Design review of the part built by this model. Coordinates are the model's own, in mm. A direction names the side the tool comes from. Give positions to 0.01 mm unless a question says otherwise; leave off trailing zeros. Write each loop counter-clockwise with the first axis right and the second up, starting at its lowest first coordinate (ties: lowest second). Pieces come first, ordered by that corner, then holes. Notation, with made-up numbers: (36, -38) - (90, -38) arc R11 cw to (90, -28) - close; hole circle Ø6 at (-37.75, 57). An arc over 180 degrees is marked (long way). Use a Markdown table: item, result. Add a question column.
```python
from build123d import *

# Parameters (mm, degrees)
SKETCH1_W           = 61
SKETCH1_H           = 61
SKETCH1_W_2         = 57
SKETCH1_H_2         = 57
BOSS_EXTRUDE2_DEPTH = 30
SKETCH2_W           = 58.6
SKETCH2_H           = 58.6
CUT_EXTRUDE1_DEPTH  = 3.2
SKETCH4_RX          = 3
SKETCH4_RY          = 2.5
CUT_EXTRUDE2_DEPTH  = 73.878323252
SKETCH5_W           = 57
SKETCH5_H           = 57
BOSS_EXTRUDE3_DEPTH = 2


with BuildPart() as part:
    # Sketch1 → Boss-Extrude2 (new body)
    with BuildSketch(Plane(origin=(0, 0, 0), x_dir=(1, 0, 0), z_dir=(0, 1, 0))):
        with Locations((0, 28.5)):
            Rectangle(SKETCH1_W, SKETCH1_H)
        with Locations((0, 28.5)):
            Rectangle(SKETCH1_W_2, SKETCH1_H_2, mode=Mode.SUBTRACT)
    extrude(amount=BOSS_EXTRUDE2_DEPTH)

    # Sketch2 → Cut-Extrude1 (cut)
    with BuildSketch(Plane(origin=(0, 30, 0), x_dir=(1, 0, 0), z_dir=(0, 1, 0))):
        with Locations((0, 28.5)):
            Rectangle(SKETCH2_W, SKETCH2_H)
    extrude(amount=-CUT_EXTRUDE1_DEPTH, mode=Mode.SUBTRACT)

    # Sketch4 → Cut-Extrude2 (cut, through all)
    with BuildSketch(Plane(origin=(0, 0, 0), x_dir=(-1, 0, 0), z_dir=(0, 0, -1))):
        with BuildLine():
            Line((-5.98277454, 23.2), (-5.98277454, 25.8))
            Line((-5.98277454, 25.8), (-8.131556664, 25.8))
            ThreePointArc((-8.131556664, 25.8), (-8.523646049, 25.719927124), (-8.852943985, 25.492531828))
            Line((-8.852943985, 25.492531828), (-9.479161861, 24.840221541))
            ThreePointArc((-9.479161861, 24.840221541), (-9.685510311, 24.520927357), (-9.75777454, 24.147689712))
            Line((-9.75777454, 24.147689712), (-9.75777454, 23.6))
            ThreePointArc((-9.75777454, 23.6), (-9.640617252, 23.317157288), (-9.35777454, 23.2))
            Line((-9.35777454, 23.2), (-5.98277454, 23.2))
        make_face()
        with BuildLine():
            Line((-3.833992416, 25.8), (-5.98277454, 25.8))
            Line((-5.98277454, 25.8), (-5.98277454, 23.2))
            Line((-5.98277454, 23.2), (-2.60777454, 23.2))
            ThreePointArc((-2.60777454, 23.2), (-2.324931828, 23.317157288), (-2.20777454, 23.6))
            Line((-2.20777454, 23.6), (-2.20777454, 24.147689712))
            ThreePointArc((-2.20777454, 24.147689712), (-2.280038769, 24.520927357), (-2.486387219, 24.840221541))
            Line((-2.486387219, 24.840221541), (-3.112605095, 25.492531828))
            ThreePointArc((-3.112605095, 25.492531828), (-3.441903031, 25.719927124), (-3.833992416, 25.8))
        make_face()
        with Locations(Location((5.992555786, 23.215339324), (0, 0, 180))):
            Ellipse(SKETCH4_RX, SKETCH4_RY)
    extrude(amount=-CUT_EXTRUDE2_DEPTH, mode=Mode.SUBTRACT)

    # Sketch5 → Boss-Extrude3 (add)
    with BuildSketch(Plane.XZ):
        with Locations((0, -28.5)):
            Rectangle(SKETCH5_W, SKETCH5_H)
    extrude(amount=-BOSS_EXTRUDE3_DEPTH)


solid = part.part
```
(1) Add section D-D (y = 28). State the section outline as (x, z) points, and give its area (3 significant figures).
(2) For line 1 along Z through (x, y) = (16, 26); line 2 along X through (y, z) = (8.5, -16.5); line 3 along Z through (x, y) = (-1, 28), list the stretches that pass through material, from the lowest coordinate up.
(3) Tool access review of faces 1 (the face through (6, 23.2, 1)), 2 (the face through (0, 14, -57)), 3 (the face through (30.5, 15, -28)): name each direction out of +Z, -Z, +X, -X, +Y, -Y from which nothing blocks a thin tool from reaching the whole face with its end or side.
(4) Mouldability with a two-part tool opening along Z and no side actions: class faces 4 (the face through (28.5, 14, -28)), 5 (the face through (0, 15, -59)), 6 (the face through (6, 25.8, 1)) as +Z half, -Z half, draft (parallel to the pull), parting line (faces both ways), or undercut.
(5) Add section B-B (x = -23). State the section outline as (y, z) points.
(6) Add section C-C (z = -49.5). State the section outline as (x, y) points, and give its area (3 significant figures).
(7) Insertion check: pin 1 (8 mm diameter, centred on x = -9, z = -45, fed in from +Y). The pin has a flat end and moves straight along its axis. Give the tip position at first contact, or say it passes through.
(8) Add section A-A (y = 8). State the section outline as (x, z) points, and give its area (3 significant figures).
Answers follow:
| question | item | result |
|---|---|---|
| 1 | outline | (-30.5, -59) - (30.5, -59) - (30.5, 2) - (-30.5, 2) - close; hole (-29.3, -57.8) - (29.3, -57.8) - (29.3, 0.8) - (-29.3, 0.8) - close |
| 1 | area | 287 mm^2 |
| 2 | line 1 | -59 to -57, 0 to 2 |
| 2 | line 2 | -30.5 to -28.5, 28.5 to 30.5 |
| 2 | line 3 | -59 to -57.8, 0.8 to 2 |
| 3 | face 1 | +Z |
| 3 | face 2 | +Y |
| 3 | face 3 | +Z, -Z, +X, +Y, -Y |
| 4 | face 4 | undercut |
| 4 | face 5 | -Z half |
| 4 | face 6 | draft |
| 5 | outline | (0, -59) - (30, -59) - (30, -57.8) - (26.8, -57.8) - (26.8, -57) - (2, -57) - (2, 0) - (26.8, 0) - (26.8, 0.8) - (30, 0.8) - (30, 2) - (0, 2) - close |
| 6 | outline | (-30.5, 0) - (30.5, 0) - (30.5, 30) - (29.3, 30) - (29.3, 26.8) - (28.5, 26.8) - (28.5, 2) - (-28.5, 2) - (-28.5, 26.8) - (-29.3, 26.8) - (-29.3, 30) - (-30.5, 30) - close |
| 6 | area | 229 mm^2 |
| 7 | pin 1 | y = 2 |
| 8 | outline | (-30.5, -59) - (30.5, -59) - (30.5, 2) - (-30.5, 2) - close; hole (-28.5, -57) - (28.5, -57) - (28.5, 0) - (-28.5, 0) - close |
| 8 | area | 472 mm^2 |
